Read the model definition and answer for the solid it produces. Units are mm, in the model's axes. Face numbers are marked on the shaded views. A direction names the side the tool comes from. Give positions to 0.01 mm unless a question says otherwise; leave off trailing zeros. Loops run counter-clockwise (first coordinate to the right, second up) from the corner with the lowest first, then second, coordinate; pieces in that order, holes last. Notation, with made-up numbers: (15, 75.5) - (74, 75.5) arc R7 cw to (74, 81.5) - close; hole circle Ø8 at (29, 29.5). An arc over 180 degrees is marked (long way). Write item = value, one per line.
```python
from build123d import *

# Parameters (mm, degrees)
F0_W     = 101.406738162
F0_H     = 103.0912548304
F0_W_2   = 74.2010474205
F0_H_2   = 78.1673192978
F1_DEPTH = 38.1
F2_W     = 13.6028453708
F2_H     = 56.0740102082
F3_DEPTH = 25.4
F2_H_2   = 53.0724562705
F4_DEPTH = 25.4
F5_R     = 12.4226697252
F6_DEPTH = 25.4
F7_R     = 11.7834333481
F8_DEPTH = 25.4


with BuildPart() as f1:
    # F0 (on Top) → F1 (new body)
    with BuildSketch(Plane.XY):
        Rectangle(F0_W, F0_H)
        Rectangle(F0_W_2, F0_H_2, mode=Mode.SUBTRACT)
    extrude(amount=F1_DEPTH)

    # F2 (on face) → F3 (cut)
    with BuildSketch(Plane.XY.offset(38.1)):
        with Locations((-43.9019463956, 1.6720136628)):
            Rectangle(F2_W, F2_H)
    extrude(amount=-F3_DEPTH, mode=Mode.SUBTRACT)

    # F2 (on face) → F4 (cut)
    with BuildSketch(Plane.XY.offset(38.1)):
        with Locations((43.9019463956, -0.9162034839)):
            Rectangle(F2_W, F2_H_2)
    extrude(amount=-F4_DEPTH, mode=Mode.SUBTRACT)

    # F5 (on face) → F6 (cut)
    with BuildSketch(Plane.XZ.offset(51.5456274152)):
        with Locations((0, 17.6801010966)):
            Circle(F5_R)
    extrude(amount=-F6_DEPTH, mode=Mode.SUBTRACT)

    # F7 (on face) → F8 (cut)
    with BuildSketch(Plane(origin=(0, 51.5456274152, 0), x_dir=(-1, 0, 0), z_dir=(0, 1, 0))):
        with Locations((0, 16.2762645632)):
            Circle(F7_R)
    extrude(amount=-F8_DEPTH, mode=Mode.SUBTRACT)


solid = f1.part
```
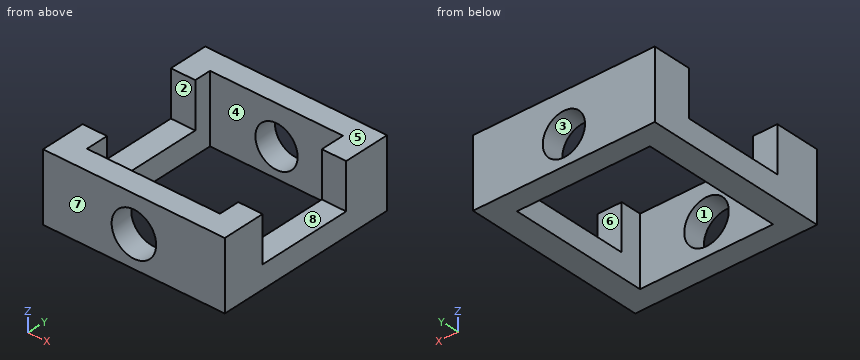
1) A cutting plane is placed at B-B on y = 3. Determine the outline of the cut face in (x, z).
Output:
outline = (-50.7, 0) - (-37.1, 0) - (-37.1, 12.7) - (-50.7, 12.7) - close; (37.1, 0) - (50.7, 0) - (50.7, 12.7) - (37.1, 12.7) - close
2) Each of these flat-tipped pins is pushed along its axis until it touches: P1, Ø7, axis at x = -42, y = 8, coming from the +Z side; P2, Ø6, axis at y = 18.5, z = 15, coming from the +X side. Where does it stop, or does it pass through?
Output:
P1 = 12.7
P2 = 50.7
3) The mould has two halves that part along Y. Classify the marked faces 5, 6, 7 and 8: pulls with the +Y half, pulls with the -Y half, needs draft (parallel to the pull), parting line crosses it, or undercut.
Output:
face_5 = needs draft
face_6 = undercut
face_7 = pulls with the -Y half
face_8 = undercut
4) A cutting plane is placed at C-C on z = 34.5. Determine the outline of the cut face in (x, y) (3 decimals), then the cut area to 3 significant figures.
Output:
outline = (-50.703, -51.546) - (50.703, -51.546) - (50.703, -27.452) - (37.101, -27.452) - (37.101, -39.084) - (-37.101, -39.084) - (-37.101, -26.365) - (-50.703, -26.365) - close; (-50.703, 29.709) - (-37.101, 29.709) - (-37.101, 39.084) - (37.101, 39.084) - (37.101, 25.62) - (50.703, 25.62) - (50.703, 51.546) - (-50.703, 51.546) - close
area = 3,170 mm²
5) A cutting plane is placed at A-A on x = 0. Determine the outline of the cut face in (y, z), then the cut area to 3 significant figures.
Output:
outline = (-51.55, 0) - (-39.08, 0) - (-39.08, 5.26) - (-51.55, 5.26) - close; (-51.55, 30.1) - (-39.08, 30.1) - (-39.08, 38.1) - (-51.55, 38.1) - close; (39.08, 0) - (51.55, 0) - (51.55, 4.49) - (39.08, 4.49) - close; (39.08, 28.06) - (51.55, 28.06) - (51.55, 38.1) - (39.08, 38.1) - close
area = 346 mm²
6) Find the intervals of material crossed by probe 1 along Y at (x, z) = (38, 32); probe 2 along X at (y, z) = (-5.5, 6); probe 3 along Y at (x, z) = (-21, 9.5), in increasing order.
Output:
probe_1 = -51.55 to -27.45, 25.62 to 51.55
probe_2 = -50.7 to -37.1, 37.1 to 50.7
probe_3 = -51.55 to -39.08, 39.08 to 51.55
7) A cutting plane is placed at D-D on x = -27.5. Determine the outline of the cut face in (y, z), then the cut area to 3 significant figures.
Output:
outline = (-51.55, 0) - (-39.08, 0) - (-39.08, 38.1) - (-51.55, 38.1) - close; (39.08, 0) - (51.55, 0) - (51.55, 38.1) - (39.08, 38.1) - close
area = 950 mm²
8) A tool of negligible diameter and unlimited length cuts with its end or side. For the marked faces 1, 2, 3 and 4, from which of +Z, -Z, +X, -X, +Y, -Y can it reach the whole face along a straight path? Write none if from no direction.
Output:
face_1 = -Y
face_2 = +Z, -X
face_3 = +Y
face_4 = +Z, -Z
